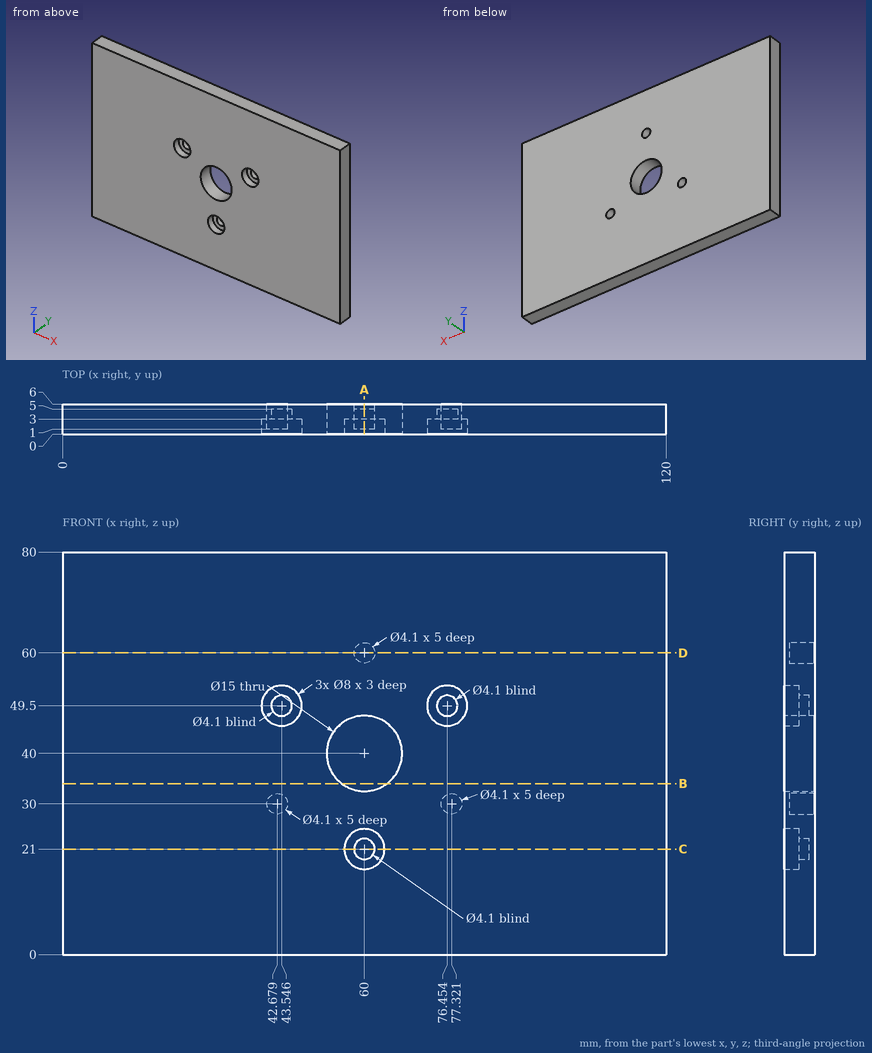
Study the drawing (mm; zero at the part's minimum x, y, z) and answer. Coordinates: 2 decimals unless noted, no trailing zeros. Write each loop counter-clockwise with the first axis right and the second up, starting at its lowest first coordinate (ties: lowest second). Pieces come first, ordered by that corner, then holes. Notation, with made-up numbers: (13, 41.5) - (43, 41.5) arc R27 cw to (43, 71.5) - close; hole circle Ø3 at (1, -26.75). An arc over 180 degrees is marked (long way). One line per item, written item: value.
1) Find section D-D (z = 60). Give the vertices of the cut face in (x, y).
Geometry check:
outline: (0, 0) - (120, 0) - (120, 6) - (62.05, 6) - (62.05, 1) - (57.95, 1) - (57.95, 6) - (0, 6) - close
2) Find section B-B (z = 34). Give the vertices of the cut face in (x, y), and give its area (3 significant figures).
Geometry check:
outline: (0, 0) - (55.5, 0) - (55.5, 6) - (0, 6) - close; (64.5, 0) - (120, 0) - (120, 6) - (64.5, 6) - close
area: 666 mm2
3) Each of these flat-tipped pins is pushed along its axis until it touches: pin 1 Ø3.5 at (x, z) = (42.68, 30) entering from +Y; pin 2 Ø4 at (x, z) = (60, 19.5) entering from -Y; pin 3 Ø2 at (x, z) = (44, 50) entering from -Y. Where does it stop, or does it pass through?
Geometry check:
pin 1: stops at y = 1
pin 2: stops at y = 3
pin 3: stops at y = 5
4) Find section C-C (z = 21). Give the vertices of the cut face in (x, y), and give its area (3 significant figures).
Geometry check:
outline: (0, 0) - (56, 0) - (56, 3) - (57.95, 3) - (57.95, 5) - (62.05, 5) - (62.05, 3) - (64, 3) - (64, 0) - (120, 0) - (120, 6) - (0, 6) - close
area: 688 mm2
5) Find section A-A (x = 60). Give the vertices of the cut face in (y, z).
Geometry check:
outline: (0, 0) - (6, 0) - (6, 32.5) - (0, 32.5) - (0, 25) - (3, 25) - (3, 23.05) - (5, 23.05) - (5, 18.95) - (3, 18.95) - (3, 17) - (0, 17) - close; (0, 47.5) - (6, 47.5) - (6, 57.95) - (1, 57.95) - (1, 62.05) - (6, 62.05) - (6, 80) - (0, 80) - close
6) Consider line 1 along X through (y, z) = (0.95, 49.5) (1 decimal); line 2 along X through (y, z) = (4.1, 21); line 3 along X through (y, z) = (2.2, 21). Determine where each line is inside the solid, lowest interval first. Write a range as from..to.
Geometry check:
line 1: x = 0..39.5, 47.5..72.5, 80.5..120
line 2: x = 0..57.95, 62.05..120
line 3: x = 0..56, 64..120
